For this review, take the finished solid that the model builds, in its own axes (mm). A direction names the side the tool comes from. Round coordinates to 2 decimals unless told otherwise and drop trailing zeros. Order: outer loops, then holes, each group sorted by start corner. A loop starts at its lowest first (then second) coordinate and runs counter-clockwise, first axis right, second up. Notation, with made-up numbers: (33, -7.75) -> (71, -7.75) arc R18 cw to (71, 2.25) -> close; hole circle Ø6 at (-4.5, -32). An arc over 180 degrees is marked (long way). Use a Markdown table: item, result. Add a question column.
1) Clearance check with flat-ended pins moving along their axes: P1, Ø4, axis at y = -82.5, z = -74, coming from the +X side; P2, Ø3, axis at y = -55, z = 18.5, coming from the +X side. State where each tip first meets the part, or that it passes through.
2) Consider section A-A (y = -127). State the section outline as (x, z) points, plus the area to 3 significant figures.
3) Draft analysis for pull direction Y (two halves, no side actions). For faces 3 (the face through (-27, -279.4, 2)), 4 (the face through (75.844, -290, 2.134)), 5 (the face through (-30, -304.8, 2)), 6 (the face through (-47.003, -29.219, 123.724)), state which applies: pulls with the +Y half, pulls with the -Y half, needs draft (parallel to the pull), parting line crosses it, or undercut.
4) Wall thickness on line 1 along Z through (x, y) = (15, -198.5); line 2 along Y through (x, z) = (-35.5, 89.5); line 3 along Z through (x, y) = (89, -162): over which ranges is each line inside the solid? List them lowest first. Write a range as [from, to].
5) Consider section B-B (z = 41). State the section outline as (x, y) points, plus the area to 3 significant figures.
6) Machinability: for faces 1 (the face through (-126.7, -154.2, -1.8)), 2 (the face through (-27, -151, -152.4)), which of the approach directions +Z, -Z, +X, -X, +Y, -Y give a long, thin tool a straight path to every point of the face, cutting with its end or side? Answer none if there is none.
```python
from build123d import *

# Parameters (mm, degrees)
F0_W        = 304.8
F0_H        = 304.8
F1_DEPTH    = 304.8
F3_DEPTH    = 304.801
F4_T1_DEPTH = 393.7
F4_T3_DEPTH = 444.5
F5_W        = 254
F5_H        = 258.2043365391
F7_R        = 12.7


# Not quite as in the source:
# - a fillet or chamfer that OpenCascade refuses, or shapes differently, is made with other operations: its cross-section is extruded or revolved along the edge and cut away or added


with BuildPart() as f1:
    # F0 (on Front) → F1 (new body)
    with BuildSketch(Plane.XZ):
        Rectangle(F0_W, F0_H)
    extrude(amount=F1_DEPTH)

    # F2 (on face) → F3 (cut, through all)
    with BuildSketch(Plane.XZ.offset(304.8)):
        Polygon((152.4, 152.4), (50.8, 152.4), (101.6, -152.4), (152.4, -152.4), align=None)
    extrude(amount=-F3_DEPTH, mode=Mode.SUBTRACT)

    # F4: fillet of radius 38.1 on 4 edges, made by hand

    # F4_s2 → F4_t1 (cut)
    with BuildSketch(Plane.YZ.offset(-247.65)):
        with BuildLine():
            add(Edge.make_bspline(
                [(-266.7, 152.4), (-304.8, 152.4), (-304.8, 114.3)],
                knots=[0, 0, 0, 1, 1, 1], degree=2, weights=[1, 1, 1]))
            Line((-304.8, 114.3), (-304.8, 152.4))
            Line((-304.8, 152.4), (-266.7, 152.4))
        make_face()
        with BuildLine():
            add(Edge.make_bspline(
                [(-38.1, 152.4), (0, 152.4), (0, 114.3)],
                knots=[0, 0, 0, 1, 1, 1], degree=2, weights=[1, 1, 1]))
            Line((0, 114.3), (0, 152.4))
            Line((0, 152.4), (-38.1, 152.4))
        make_face()
    extrude(amount=F4_T1_DEPTH, mode=Mode.SUBTRACT)

    # F4_s4 → F4_t3 (cut)
    with BuildSketch(Plane.YZ.offset(-247.65)):
        with BuildLine():
            add(Edge.make_bspline(
                [(0, -114.3), (0, -152.4), (-38.1, -152.4)],
                knots=[0, 0, 0, 1, 1, 1], degree=2, weights=[1, 1, 1]))
            Line((-38.1, -152.4), (0, -152.4))
            Line((0, -152.4), (0, -114.3))
        make_face()
        with BuildLine():
            add(Edge.make_bspline(
                [(-304.8, -114.3), (-304.8, -152.4), (-266.7, -152.4)],
                knots=[0, 0, 0, 1, 1, 1], degree=2, weights=[1, 1, 1]))
            Line((-266.7, -152.4), (-304.8, -152.4))
            Line((-304.8, -152.4), (-304.8, -114.3))
        make_face()
    extrude(amount=F4_T3_DEPTH, mode=Mode.SUBTRACT)

    # F6: sweep along a path in F6_path
    with BuildLine(Plane(origin=(50.8, -266.7, 152.4), x_dir=(0, -1, 0), z_dir=(0, 0, -1))) as f6_path:
        Line((0, 0), (0, 203.2))
    # F5 (on face) → F6 (sweep, cut)
    with BuildSketch(Plane(origin=(74.1405405405, 0, 12.3567567568), x_dir=(0, 1, 0), z_dir=(0.9863939238, 0, 0.1643989873))):
        with Locations((-152.4, -12.5272028327)):
            Rectangle(F5_W, F5_H)
    sweep(path=f6_path.line, mode=Mode.SUBTRACT)

    # F7
    f7_edges = [f1.edges().sort_by_distance(p)[0] for p in [
        (-4.175734, -279.4, -127.345594),
        (-4.175734, -25.4, -127.345594),
        (-46.624266, -279.4, 127.345594),
        (-46.624266, -25.4, 127.345594),
    ]]
    fillet(f7_edges, radius=F7_R)


solid = f1.part
```
Results list:
| question | item | result |
|---|---|---|
| 1 | P1 | x = -114.33 |
| 1 | P2 | x = -129.83 |
| 2 | outline | (-152.4, -152.4) -> (101.6, -152.4) -> (97.42, -127.35) -> (-105.78, -127.35) -> (-148.22, 127.35) -> (54.98, 127.35) -> (50.8, 152.4) -> (-152.4, 152.4) -> close |
| 2 | area | 17,900 mm2 |
| 3 | face 3 | undercut |
| 3 | face 4 | needs draft |
| 3 | face 5 | pulls with the -Y half |
| 3 | face 6 | undercut |
| 4 | line 1 | [-152.4, -127.35], [127.35, 152.4] |
| 4 | line 2 | [-304.8, -279.4], [-25.4, 0] |
| 4 | line 3 | [-152.4, -127.35] |
| 5 | outline | (-152.4, -304.8) -> (69.37, -304.8) -> (69.37, -279.4) -> (-133.83, -279.4) -> (-133.83, -25.4) -> (69.37, -25.4) -> (69.37, 0) -> (-152.4, 0) -> close |
| 5 | area | 16,000 mm2 |
| 6 | face 1 | +X |
| 6 | face 2 | -Z, +X, -X, +Y, -Y |
